Read the model definition and answer for the solid it produces. Units are mm, in the model's axes. A direction names the side the tool comes from. Coordinates: 2 decimals unless noted, no trailing zeros. Write each loop counter-clockwise with the first axis right and the second up, starting at its lowest first coordinate (ties: lowest second). Pieces come first, ordered by that corner, then holes. Notation, with made-up numbers: (-33.5, 11.5) - (24.5, 11.5) arc R33 ccw to (24.5, 41.5) - close; hole circle Ø3 at (-37, 71.5). An arc over 180 degrees is marked (long way). Return JSON: item names as keys, results as strings.
```python
from build123d import *

# Parameters (mm, degrees)
F0_R     = 9.525
F1_DEPTH = 127
F2_R     = 9.525
F3_DEPTH = 60.96


with BuildPart() as f1:
    # F0 (on Front) → F1 (new body)
    with BuildSketch(Plane.XZ):
        Polygon((-28.575, -25.6290164173), (-28.575, -38.3290164173), (-9.525, -38.3290164173), (-9.525, -25.6290164173), (0, -25.6290164173), (0, 25.1709835827), (-38.1, 25.1709835827), (-38.1, -25.6290164173), align=None)
        with Locations((-19.05, 0)):
            Circle(F0_R, mode=Mode.SUBTRACT)
    extrude(amount=F1_DEPTH)

    # F2 (on Right) → F3 (cut)
    with BuildSketch(Plane.YZ):
        with BuildLine():
            ThreePointArc((-22.225, 0), (-25.0148079092, 6.7351920908), (-31.75, 9.525))
            Line((-31.75, 9.525), (-31.75, -9.525))
            ThreePointArc((-31.75, -9.525), (-25.0148079092, -6.7351920908), (-22.225, 0))
        make_face()
        with BuildLine():
            Line((-31.75, -9.525), (-31.75, 9.525))
            ThreePointArc((-31.75, 9.525), (-41.275, 0), (-31.75, -9.525))
        make_face()
        with Locations((-94.0945148468, -0.607660502)):
            Circle(F2_R)
    extrude(amount=-F3_DEPTH, mode=Mode.SUBTRACT)


solid = f1.part
```
(1) Flat-ended cylindrical pins translate along their axes: P1, Ø5, axis at x = -5, y = -56.5, coming from the -Z side; P2, Ø3, axis at x = -33, z = 3, coming from the +Y side; P3, Ø4, axis at y = -84.5, z = -29, coming from the -X side (3 decimals). Find the tip coordinate at first contact, or state that the pin passes through.
Answer:
{"P1": "z = -25.63", "P2": "y = 0", "P3": "x = -28.575"}
(2) A cutting plane is placed at B-B (z = 5). Determine the outline of the cut face in (x, y), and give its area (3 significant figures).
Answer:
{"outline": "(-38.1, -127) - (-27.16, -127) - (-27.16, -101.79) - (-38.1, -101.79) - close; (-38.1, -86.4) - (-27.16, -86.4) - (-27.16, -39.86) - (-38.1, -39.86) - close; (-38.1, -23.64) - (-27.16, -23.64) - (-27.16, 0) - (-38.1, 0) - close; (-10.94, -127) - (0, -127) - (0, -101.79) - (-10.94, -101.79) - close; (-10.94, -86.4) - (0, -86.4) - (0, -39.86) - (-10.94, -39.86) - close; (-10.94, -23.64) - (0, -23.64) - (0, 0) - (-10.94, 0) - close", "area": "2,090 mm²"}
(3) Which of the six approach directions +Z, -Z, +X, -X, +Y, -Y give full straight-line access (tool end or side, diameter ignored) to faces 4 (the face through (-28.575, -63, -32)), 5 (the face through (-5, -63, -25.629)), 6 (the face through (-28, 0, -6))?
Answer:
{"face 4": "-Z, -X, +Y, -Y", "face 5": "-Z, +X, +Y, -Y", "face 6": "+Z, -Z, +X, -X, +Y"}
(4) A cutting plane is placed at A-A (y = -27). Determine the outline of the cut face in (x, z) (3 decimals), and give its area (3 significant figures).
Answer:
{"outline": "(-38.1, -25.629) - (-28.575, -25.629) - (-28.575, -38.329) - (-9.525, -38.329) - (-9.525, -25.629) - (0, -25.629) - (0, -8.256) - (-14.3, -8.256) arc R9.525 cw to (-23.8, -8.256) - (-38.1, -8.256) - close; (-38.1, 8.256) - (-23.8, 8.256) arc R9.525 cw to (-14.3, 8.256) - (0, 8.256) - (0, 25.171) - (-38.1, 25.171) - close", "area": "1,530 mm²"}
(5) Straight lines are drawn through the part: line 1 (Y direction, x = -6, z = 0) (3 decimals); line 2 (Y direction, x = -3.5, z = 3); line 3 (X direction, y = -8, z = 0) (3 decimals). For each, find the intervals that lie inside material, in ascending order. Write a range as from..to.
Answer:
{"line 1": "-127..-103.6, -84.589..-41.275, -22.225..0", "line 2": "-127..-102.91, -85.28..-40.79, -22.71..0", "line 3": "-38.1..-28.575, -9.525..0"}
(6) A cutting plane is placed at C-C (x = -23.5). Determine the outline of the cut face in (y, z) (3 decimals), and give its area (3 significant figures).
Answer:
{"outline": "(-127, -38.329) - (0, -38.329) - (0, -8.422) - (-27.3, -8.422) arc R9.525 cw to (-36.2, -8.422) - (-88.648, -8.422) arc R9.525 cw to (-99.541, -8.422) - (-127, -8.422) - close; (-127, 8.422) - (-97.127, 8.422) arc R9.525 cw to (-91.062, 8.422) - (-36.2, 8.422) arc R9.525 cw to (-27.3, 8.422) - (0, 8.422) - (0, 25.171) - (-127, 25.171) - close", "area": "5,900 mm²"}
(7) Determine the mould class of faces 1 (the face through (-9.965, -78.708, 2.861)), 2 (the face through (-38.1, -63, 0)), 3 (the face through (-33, -63, -25.629)) for opening direction X: +X half, -X half, draft (parallel to the pull), parting line (faces both ways), or undercut.
Answer:
{"face 1": "undercut", "face 2": "-X half", "face 3": "draft"}
